Drawing for the job (mm, zero at the part's lowest x, y, z). A direction names the side the tool comes from. Give positions to 0.01 mm unless a question says otherwise; leave off trailing zeros. Order: outer loops, then holes, each group sorted by start corner. A loop starts at its lowest first (then second) coordinate and runs counter-clockwise, first axis right, second up. Notation, with made-up numbers: (-12.75, -8.5) - (8.25, -8.5) arc R27 ccw to (8.25, 27.5) - close; hole circle Ø1 at (-28, 71). An arc over 180 degrees is marked (long way). Use a Markdown table: item, result.
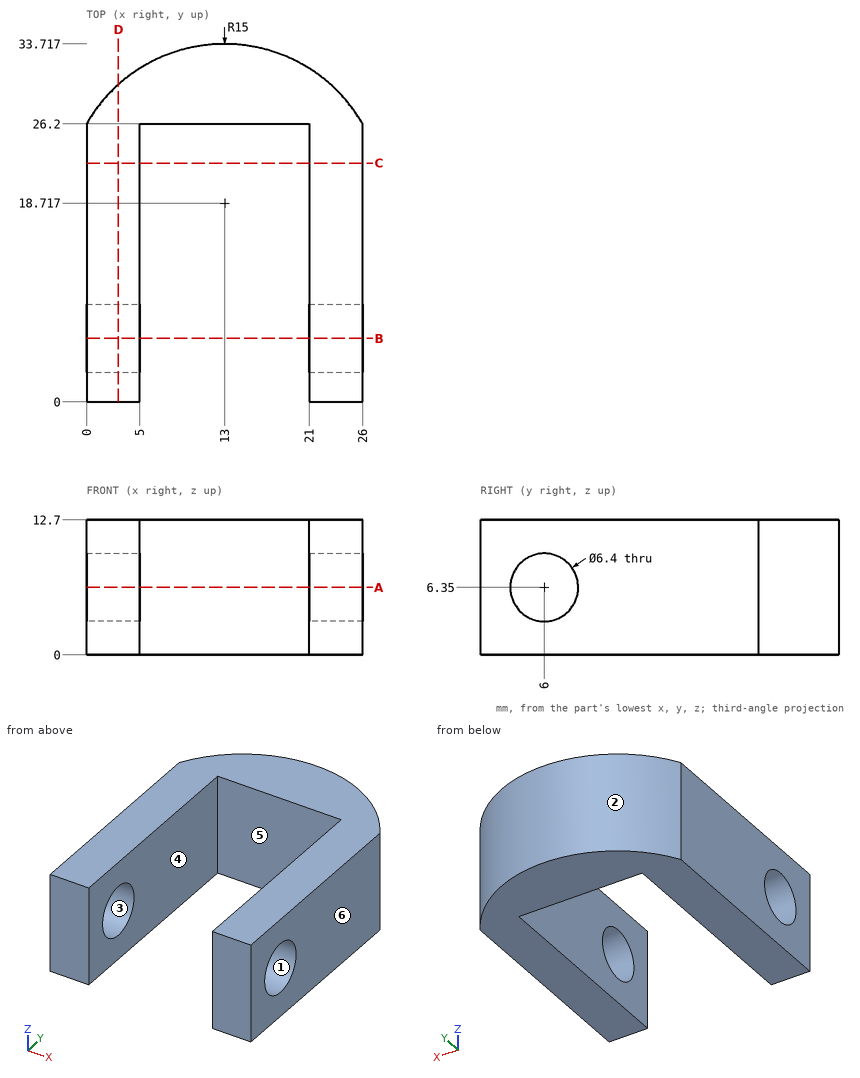
1) Two-plate mould, pull along Y, no slides. Class the marked faces 1, 2, 3 and 4: +Y half, -Y half, draft (parallel to the pull), parting line (faces both ways), or undercut.
Computed:
| item | result |
|---|---|
| face 1 | undercut |
| face 2 | +Y half |
| face 3 | undercut |
| face 4 | draft |
2) Slice it at C-C (y = 22.5). Write the cut outline in (x, z).
Computed:
| item | result |
|---|---|
| outline | (0, 0) - (5, 0) - (5, 12.7) - (0, 12.7) - close; (21, 0) - (26, 0) - (26, 12.7) - (21, 12.7) - close |
3) Slice it at D-D (x = 3). Write the cut outline in (y, z).
Computed:
| item | result |
|---|---|
| outline | (0, 0) - (29.9, 0) - (29.9, 12.7) - (0, 12.7) - close; hole circle Ø6.4 at (6, 6.35) |
4) Slice it at A-A (z = 6.35). Write the cut outline in (x, y), and give its area (3 significant figures).
Computed:
| item | result |
|---|---|
| outline | (0, 0) - (5, 0) - (5, 2.8) - (0, 2.8) - close; (0, 9.2) - (5, 9.2) - (5, 26.2) - (21, 26.2) - (21, 9.2) - (26, 9.2) - (26, 26.2) arc R15 ccw to (0, 26.2) - close; (21, 0) - (26, 0) - (26, 2.8) - (21, 2.8) - close |
| area | 337 mm² |
5) Tool access for the marked faces 5 and 6: list every direction of +Z, -Z, +X, -X, +Y, -Y with a clear straight run to the whole face (end or side of a thin tool).
Computed:
| item | result |
|---|---|
| face 5 | +Z, -Z, -Y |
| face 6 | +Z, -Z, +X, +Y, -Y |
6) Slice it at B-B (y = 6). Write the cut outline in (x, z).
Computed:
| item | result |
|---|---|
| outline | (0, 0) - (5, 0) - (5, 3.15) - (0, 3.15) - close; (0, 9.55) - (5, 9.55) - (5, 12.7) - (0, 12.7) - close; (21, 0) - (26, 0) - (26, 3.15) - (21, 3.15) - close; (21, 9.55) - (26, 9.55) - (26, 12.7) - (21, 12.7) - close |
7) Pin check, flat tips, straight feed: P1, Ø2, axis at x = 17, z = 5.5, coming from the +Y side; P2, Ø1.5, axis at x = 5.5, z = 8.5, coming from the +Y side; P3, Ø3, axis at x = 16.5, z = 3, coming from the +Y side. Stop position of each tip, or through.
Computed:
| item | result |
|---|---|
| P1 | stops at y = 33.41 |
| P2 | stops at y = 32.11 |
| P3 | stops at y = 33.58 |
8) Wall check: line 1 (X direction, y = 17.5, z = 8); line 2 (Y direction, x = 22.25, z = 6.35) (1 decimal); line 3 (Y direction, x = 22.4, z = 6.35) (1 decimal). Give the ranges that are in metal, low to high. Write a range as from..to.
Computed:
| item | result |
|---|---|
| line 1 | x = 0..5, 21..26 |
| line 2 | y = 0..2.8, 9.2..30.5 |
| line 3 | y = 0..2.8, 9.2..30.4 |
